from build123d import *

# Parameters (mm, degrees)
F2_R     = 2.54
F3_R     = 1.27
F4_R     = 2.54
F5_DEPTH = 7.62


with BuildPart() as f1:
    # F0 (on Front) → F1 (revolve)
    with BuildSketch(Plane.XZ):
        Polygon((0, 11.619149), (-12.7, 11.619149), (-12.7, 6.539149), (-6.479921, 5.224574), (-5.08, 0), (0, 0), align=None)
    revolve(axis=Axis((0, 0, 5.809575), (0, 0, 1)))

    # F2
    f2_edges = [f1.edges().sort_by_distance(p)[0] for p in [
        (6.479921, 0, 5.224574),
    ]]
    fillet(f2_edges, radius=F2_R)

    # F3
    f3_edges = [f1.edges().sort_by_distance(p)[0] for p in [
        (12.7, 0, 11.619149),
        (12.7, 0, 6.539149),
    ]]
    fillet(f3_edges, radius=F3_R)

    # F4 (on face) → F5 (cut)
    with BuildSketch(Plane(origin=(0, 0, 0), x_dir=(1, 0, 0), z_dir=(0, 0, -1))):
        Circle(F4_R)
    extrude(amount=-F5_DEPTH, mode=Mode.SUBTRACT)


solid = f1.part
For this review, take the finished solid that the model builds, in its own axes (mm). A direction names the side the tool comes from. Round coordinates to 2 decimals unless told otherwise and drop trailing zeros. Write each loop counter-clockwise with the first axis right and the second up, starting at its lowest first coordinate (ties: lowest second). Pieces come first, ordered by that corner, then holes. Notation, with made-up numbers: M 62,9.25 L 111,9.25 A25 cw 111,28.25 Z; hole C -13,61 d6. An arc over 180 degrees is marked long. Write item = value, one per line. Start each with the question number.
(1) Clearance check with flat-ended pins moving along their axes: pin 1 Ø6 at (y, z) = (-0.5, 6) entering from +X; pin 2 Ø2 at (x, z) = (1.5, 2.5) entering from -Y; pin 3 Ø6 at (y, z) = (6, 7.5) entering from -X; pin 4 Ø1 at (x, z) = (1, 6) entering from -Y. State where each tip first meets the part, or that it passes through.
(2) For line 1 along Y through (x, z) = (0, 4); line 2 along Y through (x, z) = (1, 7); line 3 along X through (y, z) = (0, 3.25), list the stretches that pass through material, from the lowest coordinate up.
(3) We need section B-B (z = 3). Give the boundary of the cut face in (x, y), then the cut area to 3 significant figures.
(4) We need section A-A (z = 1.5). Give the boundary of the cut face in (x, y), then the cut area to 3 significant figures.
(5) For faces 1 (the face through (-0.33, -2.52, 3.76)), 2 (the face through (-12.114, -3.815, 8.94)), list the 3-axis set-ups (+Z, -Z, +X, -X, +Y, -Y) from which the entire face can be reached by the end or side of a thin tool; tool diameter is ignored.
(6) The part is to be moulded in two halves that separate along Y. For faces 3 (the face through (1.065, -8.114, 5.585)), 4 (the face through (0, 0, 7.62)), 5 (the face through (-2, 2, 0)), say which applies: +Y half, -Y half, draft (parallel to the pull), parting line (faces both ways), or undercut.
Results found:
q1.pin_1 = 12.7
q1.pin_2 = -5.9
q1.pin_3 = -12.34
q1.pin_4 = -12.08
q2.line_1 = -6.17 to -2.54, 2.54 to 6.17
q2.line_2 = -12.53 to -2.33, 2.33 to 12.53
q2.line_3 = -5.95 to -2.54, 2.54 to 5.95
q3.outline = C 0,0 d11.77; hole C 0,0 d5.08
q3.area = 88.5 mm²
q4.outline = C 0,0 d10.96; hole C 0,0 d5.08
q4.area = 74.1 mm²
q5.face_1 = -Z
q5.face_2 = +Z, -Z
q6.face_3 = parting line
q6.face_4 = undercut
q6.face_5 = draft
